Can you work these out from the model? Positions are in its coordinate system, mm. A direction names the side the tool comes from. Give positions to 0.01 mm unless a question says otherwise; leave off trailing zeros. Loops run counter-clockwise (first coordinate to the right, second up) from the corner with the lowest first, then second, coordinate; pieces in that order, holes last.
from build123d import *

# Parameters (mm, degrees)
SKETCH1_W           = 30
SKETCH1_H           = 30
SKETCH1_R           = 2
BOSS_EXTRUDE1_DEPTH = 4
SKETCH2_W           = 30
SKETCH2_H           = 4
BOSS_EXTRUDE2_DEPTH = 150
CUT_EXTRUDE1_DEPTH  = 166.728693955


with BuildPart() as part:
    # Sketch1 → Boss-Extrude1 (new body)
    with BuildSketch(Plane(origin=(0, 0, 0), x_dir=(1, 0, 0), z_dir=(0, 1, 0))):
        Rectangle(SKETCH1_W, SKETCH1_H)
        with Locations(Location((0, 0, 0), (0, 0, 270))):
            Circle(SKETCH1_R, mode=Mode.SUBTRACT)
    extrude(amount=BOSS_EXTRUDE1_DEPTH)

    # Sketch2 → Boss-Extrude2 (add)
    with BuildSketch(Plane(origin=(0, 0, -15), x_dir=(-1, 0, 0), z_dir=(0, 0, -1))):
        with Locations((0, 2)):
            Rectangle(SKETCH2_W, SKETCH2_H)
    extrude(amount=BOSS_EXTRUDE2_DEPTH)

    # Sketch3 → Cut-Extrude1 (cut, through all)
    with BuildSketch(Plane(origin=(0, 4, 0), x_dir=(1, 0, 0), z_dir=(0, 1, 0))):
        with BuildLine():
            Line((-3, 10), (-3, 160))
            ThreePointArc((-3, 160), (0, 163), (3, 160))
            Line((3, 160), (3, 10))
            ThreePointArc((3, 10), (0, 7), (-3, 10))
        make_face()
    extrude(amount=-CUT_EXTRUDE1_DEPTH, mode=Mode.SUBTRACT)


solid = part.part
(1) Which directions (+Z, -Z, +X, -X, +Y, -Y) give clear straight access to the entire face, cutting with the end or side of a thin tool? Please do faces 1 (the flat face through (4, 0, -74)), 2 (the cylindrical face through (0, 2, -163)).
Returned:
face 1: +Z, -Z, +X, -X, -Y
face 2: +Y, -Y
(2) Suppose I cut it at B-B on x = 0. List the corners of the cut face in (y, z) for me.
Returned:
outline: (0, -165) - (4, -165) - (4, -163) - (0, -163) - close; (0, -7) - (4, -7) - (4, -2) - (0, -2) - close; (0, 2) - (4, 2) - (4, 15) - (0, 15) - close
(3) Thinking about a two-plate mould opening in X: for faces 3 (the flat face through (15, 2, -74)), 4 (the flat face through (0, 2, -165)), 5 (the flat face through (-3, 2, -84)), which applies, pulls with the +X half, pulls with the -X half, needs draft (parallel to the pull), parting line crosses it, or undercut?
Returned:
face 3: pulls with the +X half
face 4: needs draft
face 5: undercut
(4) Suppose I cut it at D-D on z = -127. List the corners of the cut face in (x, y) for me, plus the area to 3 significant figures.
Returned:
outline: (-15, 0) - (-3, 0) - (-3, 4) - (-15, 4) - close; (3, 0) - (15, 0) - (15, 4) - (3, 4) - close
area: 96.0 mm2
(5) Please list where these lines run through material, in increasing order: probe 1 along X at (y, z) = (3.7, -103.5); probe 2 along X at (y, z) = (2.85, 0); probe 3 along Z at (x, y) = (-2.5, 2.5).
Returned:
probe 1: x = -15 to -3, 3 to 15
probe 2: x = -15 to -2, 2 to 15
probe 3: z = -165 to -161.66, -8.34 to 15
(6) Suppose I cut it at A-A on z = 0. List the corners of the cut face in (x, y) for me, plus the area to 3 significant figures.
Returned:
outline: (-15, 0) - (-2, 0) - (-2, 4) - (-15, 4) - close; (2, 0) - (15, 0) - (15, 4) - (2, 4) - close
area: 104 mm2
(7) Suppose I cut it at C-C on y = 2. List the corners of the cut face in (x, z) for me.
Returned:
outline: (-15, -165) - (15, -165) - (15, 15) - (-15, 15) - close; hole (-3, -160) arc R3 ccw to (3, -160) - (3, -10) arc R3 ccw to (-3, -10) - close; hole circle Ø4 at (0, 0)
